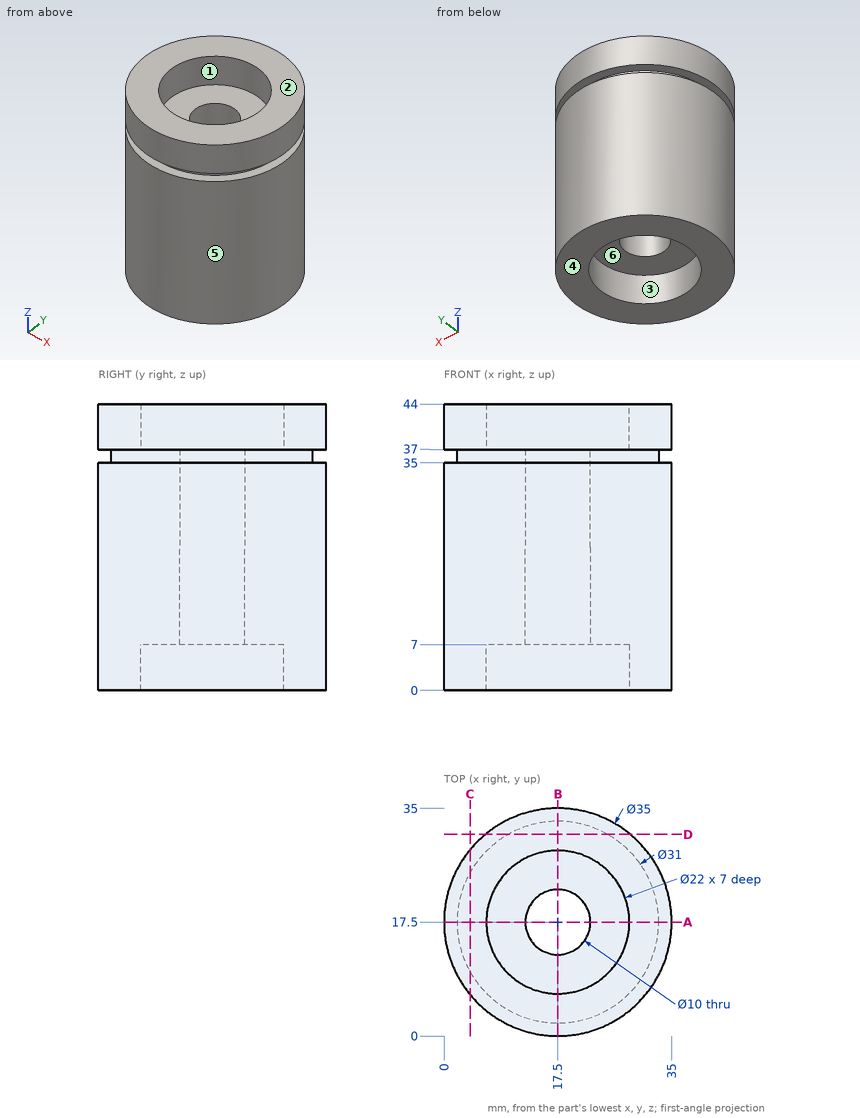
Here's the drawing with two shaded views (mm, measured from the low corner). I have some questions. A direction names the side the tool comes from. Give positions to 0.01 mm unless a question says otherwise; leave off trailing zeros. Loops run counter-clockwise (first coordinate to the right, second up) from the corner with the lowest first, then second, coordinate; pieces in that order, holes last. Notation, with made-up numbers: (-8.5, 47) -> (10.5, 47) arc R26 ccw to (10.5, 75) -> close; hole circle Ø4 at (45, 2.5). An arc over 180 degrees is marked (long way). Use one line per item in the form item = value.
1) For the marked faces 1, 2 and 3, which set-ups out of +Z, -Z, +X, -X, +Y, -Y let a thin tool reach every point of the face, with its end or its side?
Answers:
face_1 = +Z
face_2 = +Z, +X, -X, +Y, -Y
face_3 = -Z
2) If we section it at C-C (x = 4): Please give me the cut outline in (y, z).
Answers:
outline = (6.36, 0) -> (28.64, 0) -> (28.64, 35) -> (25.12, 35) -> (25.12, 37) -> (28.64, 37) -> (28.64, 44) -> (6.36, 44) -> (6.36, 37) -> (9.88, 37) -> (9.88, 35) -> (6.36, 35) -> close
3) I need wall thicknesses on line 1 along Z through (x, y) = (16, 2); line 2 along Y through (x, z) = (17.5, 3.25); line 3 along X through (y, z) = (17, 41). Which ranges of each line are inside material? Lowest first, please.
Answers:
line_1 = 0 to 35, 37 to 44
line_2 = 0 to 6.5, 28.5 to 35
line_3 = 0.01 to 6.51, 28.49 to 34.99
4) Will these pins go through, and if not, where does the flat tip stop? pin 1 (4 mm diameter, centred on y = 17, z = 33.5, fed in from -X); pin 2 (1 mm diameter, centred on x = 14.5, y = 14, fed in from +Z); pin 3 (5 mm diameter, centred on x = 14, z = 37.5, fed in from +Y); pin 4 (1 mm diameter, centred on x = 15, y = 18, fed in from -Z).
Answers:
pin_1 = 0
pin_2 = 37
pin_3 = 34.97
pin_4 = through
5) We'd pull the mould along Y, two halves only. Please class the marked faces 4, 5 and 6: released by +Y, released by -Y, zero draft, split by the parting line, or undercut.
Answers:
face_4 = zero draft
face_5 = split by the parting line
face_6 = undercut
6) If we section it at A-A (y = 17.5): Please give me the cut outline in (x, z), plus the area to 3 significant figures.
Answers:
outline = (0, 0) -> (6.5, 0) -> (6.5, 7) -> (12.5, 7) -> (12.5, 37) -> (6.5, 37) -> (6.5, 44) -> (0, 44) -> (0, 37) -> (2, 37) -> (2, 35) -> (0, 35) -> close; (22.5, 7) -> (28.5, 7) -> (28.5, 0) -> (35, 0) -> (35, 35) -> (33, 35) -> (33, 37) -> (35, 37) -> (35, 44) -> (28.5, 44) -> (28.5, 37) -> (22.5, 37) -> close
area = 924 mm²
